from build123d import *

# Parameters (mm, degrees)
SKETCH1_W              = 9.525
SKETCH1_H              = 33.3375
COMBINE1_START         = -165.1
COMBINE1_OUTLINE_R     = 6.35
COMBINE1_DEPTH         = 17.1
COMBINE1_START_2       = -168.91
COMBINE1_2_OUTLINE_R   = 5.159375
COMBINE1_2_DEPTH       = 3.81
COMBINE1_3_OUTLINE_R   = 6.35
COMBINE1_3_DEPTH       = 10.107803
COMBINE1_4_OUTLINE_R   = 6.35
COMBINE1_4_OUTLINE_R_2 = 5.159375
COMBINE1_4_DEPTH       = 3.81
COMBINE1_START_3       = 4.7625
COMBINE1_5_OUTLINE_R   = 3.571875
COMBINE1_5_OUTLINE_R_2 = 1.1303
COMBINE1_5_DEPTH       = 4.7625
COMBINE1_START_4       = -11
COMBINE1_6_OUTLINE_R   = 1.7272
COMBINE1_6_OUTLINE_R_2 = 1.1303
COMBINE1_6_DEPTH       = 15.7625
COMBINE1_START_5       = 0.793749963
COMBINE1_7_OUTLINE_R   = 2.1844
COMBINE1_7_OUTLINE_R_2 = 1.7272
COMBINE1_7_DEPTH       = 3.968750037
COMBINE1_START_6       = -33.3375
COMBINE1_8_OUTLINE_R   = 1.1303
COMBINE1_8_DEPTH       = 2.48900636


with BuildPart() as part:
    # Sketch1 → Revolve1 (revolve)
    with BuildSketch(Plane(origin=(0, 0, 0), x_dir=(1, 0, 0), z_dir=(0, 1, 0))):
        with Locations((-153.9875, 16.66875)):
            Rectangle(SKETCH1_W, SKETCH1_H)
    revolve(axis=Axis((-158.75, 0, 0), (0, 0, -1)))

    # Combine1: read off the stored shape, not the designer's step
    # Combine1 outline → Combine1 (cut)
    with BuildSketch(Plane.YZ.offset(COMBINE1_START)):
        with BuildLine():
            Line((0.79375, 0), (-0.79375, 0))
            Line((-0.79375, 0), (-0.793749936, -8.394440501))
            ThreePointArc((-0.793749936, -8.394440501), (-1e-08, -17.052925), (0.793749959, -8.394440505))
            Line((0.793749959, -8.394440505), (0.79375, 0))
        make_face()
        with Locations((0, -24.5999)):
            Circle(COMBINE1_OUTLINE_R)
    extrude(amount=COMBINE1_DEPTH, mode=Mode.SUBTRACT)

    # Combine1 2 outline → Combine1 2 (cut)
    with BuildSketch(Plane.YZ.offset(COMBINE1_START_2)):
        with BuildLine():
            Line((0.79375, 0), (-0.79375, 0))
            Line((-0.79375, 0), (-0.793749936, -8.394440501))
            ThreePointArc((-0.793749936, -8.394440501), (-1e-08, -17.052925), (0.793749959, -8.394440505))
            Line((0.793749959, -8.394440505), (0.79375, 0))
        make_face()
        with Locations((0, -24.5999)):
            Circle(COMBINE1_2_OUTLINE_R)
    extrude(amount=COMBINE1_2_DEPTH, mode=Mode.SUBTRACT)

    # Combine1 3 outline → Combine1 3 (add)
    with BuildSketch(Plane.YZ.offset(COMBINE1_START_2)):
        with BuildLine():
            Line((-0.79375, 0), (-9.525, 0))
            Line((-9.525, 0), (-9.525, -33.3375))
            Line((-9.525, -33.3375), (9.525, -33.3375))
            Line((9.525, -33.3375), (9.525, 0))
            Line((9.525, 0), (0.79375, 0))
            Line((0.79375, 0), (0.793749959, -8.394440505))
            ThreePointArc((0.793749959, -8.394440505), (-1e-08, -17.052925), (-0.793749936, -8.394440501))
            Line((-0.793749936, -8.394440501), (-0.79375, 0))
        make_face()
        with Locations((0, -24.5999)):
            Circle(COMBINE1_3_OUTLINE_R, mode=Mode.SUBTRACT)
    extrude(amount=COMBINE1_3_DEPTH)

    # Combine1 4 outline → Combine1 4 (add)
    with BuildSketch(Plane.YZ.offset(COMBINE1_START_2)):
        with Locations((0, -24.5999)):
            Circle(COMBINE1_4_OUTLINE_R)
        with Locations((0, -24.5999)):
            Circle(COMBINE1_4_OUTLINE_R_2, mode=Mode.SUBTRACT)
    extrude(amount=COMBINE1_4_DEPTH)

    # Combine1 5 outline → Combine1 5 (cut)
    with BuildSketch(Plane(origin=(0, 0, 0), x_dir=(1, 0, 0), z_dir=(0, 1, 0)).offset(COMBINE1_START_3)):
        with Locations((-158.75, 4.9911)):
            Circle(COMBINE1_5_OUTLINE_R)
        with Locations((-158.75, 24.5999)):
            Circle(COMBINE1_5_OUTLINE_R_2)
    extrude(amount=COMBINE1_5_DEPTH, mode=Mode.SUBTRACT)

    # Combine1 6 outline → Combine1 6 (cut)
    with BuildSketch(Plane(origin=(0, 0, 0), x_dir=(1, 0, 0), z_dir=(0, 1, 0)).offset(COMBINE1_START_4)):
        with Locations((-158.75, 4.9911)):
            Circle(COMBINE1_6_OUTLINE_R)
        with Locations((-158.75, 24.5999)):
            Circle(COMBINE1_6_OUTLINE_R_2)
    extrude(amount=COMBINE1_6_DEPTH, mode=Mode.SUBTRACT)

    # Combine1 7 outline → Combine1 7 (cut)
    with BuildSketch(Plane(origin=(0, 0, 0), x_dir=(1, 0, 0), z_dir=(0, 1, 0)).offset(COMBINE1_START_5)):
        with Locations((-158.75, 4.9911)):
            Circle(COMBINE1_7_OUTLINE_R)
        with Locations((-158.75, 4.9911)):
            Circle(COMBINE1_7_OUTLINE_R_2, mode=Mode.SUBTRACT)
    extrude(amount=COMBINE1_7_DEPTH, mode=Mode.SUBTRACT)

    # Combine1 8 outline → Combine1 8 (cut)
    with BuildSketch(Plane.XY.offset(COMBINE1_START_6)):
        with Locations((-158.75, 0)):
            Circle(COMBINE1_8_OUTLINE_R)
    extrude(amount=COMBINE1_8_DEPTH, mode=Mode.SUBTRACT)


solid = part.part
Model file for the job. Use its own axes, mm. A direction names the side the tool comes from. Give positions to 0.01 mm unless a question says otherwise; leave off trailing zeros. Loops run counter-clockwise (first coordinate to the right, second up) from the corner with the lowest first, then second, coordinate; pieces in that order, holes last.
1) Tool access for faces 4 (the cylindrical face through (-156.666, 2.75, -5.647)), 5 (the flat face through (-159, -0.794, -3)), 6 (the flat face through (-165.1, 0, -19)), 7 (the flat face through (-161, 0, -33.338)): list every direction of +Z, -Z, +X, -X, +Y, -Y with a clear straight run to the whole face (end or side of a thin tool).
2) Wall check: line 1 (Z direction, x = -158.75, y = 3.75); line 2 (Z direction, x = -158.75, y = -8.75); line 3 (Z direction, x = -167.65, y = 0). Give the ranges that are in metal, low to high.
3) Saw through at B-B (y = -4). Write the cut outline in (x, z).
4) Flat gauge pins, fed straight in: pin 1 Ø6 at (y, z) = (0, -24.6) entering from -X; pin 2 Ø1.5 at (x, z) = (-157.5, -9) entering from -Y; pin 3 Ø5 at (x, z) = (-158.75, -4.99) entering from +Y; pin 4 Ø5 at (y, z) = (3, -30) entering from +X. Where does each tip first touch, or does it go through?
5) Saw through at D-D (x = -153.5). Write the cut outline in (y, z), plus the area to 3 significant figures.
6) Pull direction Y, two halves, no side cores. Call faces 1 (the cylindrical face through (-159.88, 0.05, -32.11)), 2 (the flat face through (-164, -9.525, -16)), 3 (the flat face through (-159, 5, 0)): +Y half, -Y half, draft (parallel to the pull), parting line (faces both ways), or undercut.
7) Saw through at A-A (y = 0). Write the cut outline in (x, z) (1 decimal), plus the area to 3 significant figures.
Answer block:
1. face 4: +Y
1. face 5: +Z, +X, -X
1. face 6: +X
1. face 7: -Z, +X, -X, +Y, -Y
2. line 1: z = -33.34 to -29.72, -19.48 to -14.92, -10.45 to -7.18, -2.81 to 0
2. line 2: z = -33.34 to -25.73, -23.47 to -6.72, -3.26 to 0
2. line 3: z = -33.34 to -29.76, -19.44 to -17.05
3. outline: (-168.91, -33.34) - (-150.11, -33.34) - (-150.11, -29.53) - (-165.1, -29.53) - (-165.1, -27.86) - (-168.91, -27.86) - close; (-168.91, -21.34) - (-165.1, -21.34) - (-165.1, -19.67) - (-150.11, -19.67) - (-150.11, -14.44) - (-168.91, -14.44) - close; (-168.91, -10.94) - (-150.11, -10.94) - (-150.11, 0) - (-168.91, 0) - close; hole circle Ø3.45 at (-158.75, -4.99)
4. pin 1: passes through
4. pin 2: stops at y = -9.51
4. pin 3: stops at y = 4.76
4. pin 4: stops at x = -149.25
5. outline: (-7.95, -33.34) - (7.95, -33.34) - (7.95, 0) - (0.79, 0) - (0.79, -8.39) arc R4.37 cw (long way) to (-0.79, -8.39) - (-0.79, 0) - (-7.95, 0) - close; hole circle Ø12.7 at (0, -24.6)
5. area: 330 mm2
6. face 1: undercut
6. face 2: -Y half
6. face 3: draft
7. outline: (-168.9, -33.3) - (-159.9, -33.3) - (-159.9, -30.9) - (-165.1, -30.9) - (-165.1, -29.8) - (-168.9, -29.8) - close; (-168.9, -19.4) - (-165.1, -19.4) - (-165.1, -18.2) - (-149.2, -18.2) - (-149.2, -17.1) - (-168.9, -17.1) - close; (-157.6, -33.3) - (-149.2, -33.3) - (-149.2, -30.9) - (-157.6, -30.9) - close
7. area: 74.2 mm2
